```python
from build123d import *

# Parameters (mm, degrees)
BOX174_W                    = 2
BOX174_H                    = 6
BOX174_DEPTH                = 6
BOX175_W                    = 2
BOX175_H                    = 6
BOX175_DEPTH                = 6
BOX176_W                    = 2
BOX176_H                    = 6
BOX176_DEPTH                = 6
BOX173_W                    = 2
BOX173_H                    = 6
BOX173_DEPTH                = 6
CYLINDER397_R               = 1.5
CYLINDER397_DEPTH           = 100
CYLINDER398_R               = 1.5
CYLINDER398_DEPTH           = 100
CYLINDER395_R               = 1.5
CYLINDER395_DEPTH           = 100
CYLINDER396_R               = 1.5
CYLINDER396_DEPTH           = 100
CYLINDER375_R               = 1.5
CYLINDER375_DEPTH           = 50
CYLINDER375_PLACEMENT_ANGLE = 45
CYLINDER376_R               = 1.5
CYLINDER376_DEPTH           = 50
CYLINDER377_R               = 1.5
CYLINDER377_DEPTH           = 50
CYLINDER377_PLACEMENT_ANGLE = 135
CYLINDER378_R               = 1.5
CYLINDER378_DEPTH           = 50
CYLINDER379_R               = 1.5
CYLINDER379_DEPTH           = 50
CYLINDER379_PLACEMENT_ANGLE = 225
CYLINDER380_R               = 1.5
CYLINDER380_DEPTH           = 50
CYLINDER381_R               = 1.5
CYLINDER381_DEPTH           = 50
CYLINDER381_PLACEMENT_ANGLE = 45
CYLINDER374_R               = 1.5
CYLINDER374_DEPTH           = 50
BOX158_W                    = 8
BOX158_H                    = 6
BOX158_DEPTH                = 2
BOX158_PLACEMENT_ANGLE      = 45
BOX159_W                    = 8
BOX159_H                    = 6
BOX159_DEPTH                = 2
BOX160_W                    = 8
BOX160_H                    = 6
BOX160_DEPTH                = 2
BOX160_PLACEMENT_ANGLE      = 135
BOX161_W                    = 8
BOX161_H                    = 6
BOX161_DEPTH                = 2
BOX162_W                    = 8
BOX162_H                    = 6
BOX162_DEPTH                = 2
BOX162_PLACEMENT_ANGLE      = 225
BOX163_W                    = 8
BOX163_H                    = 6
BOX163_DEPTH                = 2
BOX164_W                    = 8
BOX164_H                    = 6
BOX164_DEPTH                = 2
BOX164_PLACEMENT_ANGLE      = 45
BOX157_W                    = 8
BOX157_H                    = 6
BOX157_DEPTH                = 2
CYLINDER006_R               = 3.5
CYLINDER006_DEPTH           = 16
TORUS004_R                  = 3.1
TUBE002_R                   = 54
TUBE002_R_2                 = 47
TUBE002_DEPTH               = 25


with BuildPart() as krychle174:
    # Box174 → Box174 (new body)
    with BuildSketch(Plane(origin=(32, -54, 24), x_dir=(1, 0, 0), z_dir=(0, 0, 1))):
        with Locations((1, 3)):
            Rectangle(BOX174_W, BOX174_H)
    extrude(amount=BOX174_DEPTH)


with BuildPart() as krychle175:
    # Box175 → Box175 (new body)
    with BuildSketch(Plane(origin=(38, 33, 39), x_dir=(1, 0, 0), z_dir=(0, 0, 1))):
        with Locations((1, 3)):
            Rectangle(BOX175_W, BOX175_H)
    extrude(amount=BOX175_DEPTH)


with BuildPart() as krychle176:
    # Box176 → Box176 (new body)
    with BuildSketch(Plane(origin=(38, -39, 39), x_dir=(1, 0, 0), z_dir=(0, 0, 1))):
        with Locations((1, 3)):
            Rectangle(BOX176_W, BOX176_H)
    extrude(amount=BOX176_DEPTH)


with BuildPart() as compound302:
    # Box173 → Box173 (new body)
    with BuildSketch(Plane(origin=(32, 48, 24), x_dir=(1, 0, 0), z_dir=(0, 0, 1))):
        with Locations((1, 3)):
            Rectangle(BOX173_W, BOX173_H)
    extrude(amount=BOX173_DEPTH)

    # Compound302: union Krychle174, Krychle175, Krychle176
    add(krychle174.part)
    add(krychle175.part)
    add(krychle176.part)


with BuildPart() as obj1:
    # Cylinder397 → Cylinder397 (new body)
    with BuildSketch(Plane(origin=(24, -51, 27), x_dir=(0, 0, -1), z_dir=(1, 0, 0))):
        Circle(CYLINDER397_R)
    extrude(amount=CYLINDER397_DEPTH)


with BuildPart() as obj2:
    # Cylinder398 → Cylinder398 (new body)
    with BuildSketch(Plane(origin=(34, 36, 42), x_dir=(0, 0, -1), z_dir=(1, 0, 0))):
        Circle(CYLINDER398_R)
    extrude(amount=CYLINDER398_DEPTH)


with BuildPart() as obj3:
    # Cylinder395 → Cylinder395 (new body)
    with BuildSketch(Plane(origin=(34, -36, 42), x_dir=(0, 0, -1), z_dir=(1, 0, 0))):
        Circle(CYLINDER395_R)
    extrude(amount=CYLINDER395_DEPTH)


with BuildPart() as compound303:
    # Cylinder396 → Cylinder396 (new body)
    with BuildSketch(Plane(origin=(24, 51, 27), x_dir=(0, 0, -1), z_dir=(1, 0, 0))):
        Circle(CYLINDER396_R)
    extrude(amount=CYLINDER396_DEPTH)

    # Compound303: union obj1, obj2, obj3
    add(obj1.part)
    add(obj2.part)
    add(obj3.part)


with BuildPart() as obj4:
    # Cylinder375 → Cylinder375 (new body)
    with BuildSketch(Plane.XY):
        Circle(CYLINDER375_R)
    extrude(amount=CYLINDER375_DEPTH)


with BuildPart() as obj4_1:
    # Cylinder375 placement: moved
    add(obj4.part.moved(Location((35.355339, 35.355339, -15))).rotate(Axis((35.355339, 35.355339, -15), (0, 0, 1)), CYLINDER375_PLACEMENT_ANGLE))


with BuildPart() as obj5:
    # Cylinder376 → Cylinder376 (new body)
    with BuildSketch(Plane(origin=(0, 50, -15), x_dir=(0, 1, 0), z_dir=(0, 0, 1))):
        Circle(CYLINDER376_R)
    extrude(amount=CYLINDER376_DEPTH)


with BuildPart() as obj6:
    # Cylinder377 → Cylinder377 (new body)
    with BuildSketch(Plane.XY):
        Circle(CYLINDER377_R)
    extrude(amount=CYLINDER377_DEPTH)


with BuildPart() as obj6_1:
    # Cylinder377 placement: moved
    add(obj6.part.moved(Location((-35.355339, 35.355339, -15))).rotate(Axis((-35.355339, 35.355339, -15), (0, 0, 1)), CYLINDER377_PLACEMENT_ANGLE))


with BuildPart() as obj7:
    # Cylinder378 → Cylinder378 (new body)
    with BuildSketch(Plane(origin=(-50, 0, -15), x_dir=(-1, 0, 0), z_dir=(0, 0, 1))):
        Circle(CYLINDER378_R)
    extrude(amount=CYLINDER378_DEPTH)


with BuildPart() as obj8:
    # Cylinder379 → Cylinder379 (new body)
    with BuildSketch(Plane.XY):
        Circle(CYLINDER379_R)
    extrude(amount=CYLINDER379_DEPTH)


with BuildPart() as obj8_1:
    # Cylinder379 placement: moved
    add(obj8.part.moved(Location((-35.355339, -35.355339, -15))).rotate(Axis((-35.355339, -35.355339, -15), (0, 0, 1)), CYLINDER379_PLACEMENT_ANGLE))


with BuildPart() as obj9:
    # Cylinder380 → Cylinder380 (new body)
    with BuildSketch(Plane(origin=(0, -50, -15), x_dir=(0, -1, 0), z_dir=(0, 0, 1))):
        Circle(CYLINDER380_R)
    extrude(amount=CYLINDER380_DEPTH)


with BuildPart() as obj10:
    # Cylinder381 → Cylinder381 (new body)
    with BuildSketch(Plane.XY):
        Circle(CYLINDER381_R)
    extrude(amount=CYLINDER381_DEPTH)


with BuildPart() as obj10_1:
    # Cylinder381 placement: moved
    add(obj10.part.moved(Location((35.355339, -35.355339, -15))).rotate(Axis((35.355339, -35.355339, -15), (0, 0, -1)), CYLINDER381_PLACEMENT_ANGLE))


with BuildPart() as compound298:
    # Cylinder374 → Cylinder374 (new body)
    with BuildSketch(Plane(origin=(50, 0, -15), x_dir=(1, 0, 0), z_dir=(0, 0, 1))):
        Circle(CYLINDER374_R)
    extrude(amount=CYLINDER374_DEPTH)

    # Compound298: union obj4, obj5, obj6, obj7, obj8, obj9, obj10
    add(obj4_1.part)
    add(obj5.part)
    add(obj6_1.part)
    add(obj7.part)
    add(obj8_1.part)
    add(obj9.part)
    add(obj10_1.part)


with BuildPart() as compound298_1:
    # Compound298 placement: moved
    add(compound298.part.moved(Location((0, 0, -5))))


with BuildPart() as krychle158:
    # Box158 → Box158 (new body)
    with BuildSketch(Plane.XY):
        with Locations((4, 3)):
            Rectangle(BOX158_W, BOX158_H)
    extrude(amount=BOX158_DEPTH)


with BuildPart() as krychle158_1:
    # Box158 placement: moved
    add(krychle158.part.moved(Location((34.648232, 30.405592, 23))).rotate(Axis((34.648232, 30.405592, 23), (0, 0, 1)), BOX158_PLACEMENT_ANGLE))


with BuildPart() as krychle159:
    # Box159 → Box159 (new body)
    with BuildSketch(Plane(origin=(3, 46, 23), x_dir=(0, 1, 0), z_dir=(0, 0, 1))):
        with Locations((4, 3)):
            Rectangle(BOX159_W, BOX159_H)
    extrude(amount=BOX159_DEPTH)


with BuildPart() as krychle160:
    # Box160 → Box160 (new body)
    with BuildSketch(Plane.XY):
        with Locations((4, 3)):
            Rectangle(BOX160_W, BOX160_H)
    extrude(amount=BOX160_DEPTH)


with BuildPart() as krychle160_1:
    # Box160 placement: moved
    add(krychle160.part.moved(Location((-30.405592, 34.648232, 23))).rotate(Axis((-30.405592, 34.648232, 23), (0, 0, 1)), BOX160_PLACEMENT_ANGLE))


with BuildPart() as krychle161:
    # Box161 → Box161 (new body)
    with BuildSketch(Plane(origin=(-46, 3, 23), x_dir=(-1, 0, 0), z_dir=(0, 0, 1))):
        with Locations((4, 3)):
            Rectangle(BOX161_W, BOX161_H)
    extrude(amount=BOX161_DEPTH)


with BuildPart() as krychle162:
    # Box162 → Box162 (new body)
    with BuildSketch(Plane.XY):
        with Locations((4, 3)):
            Rectangle(BOX162_W, BOX162_H)
    extrude(amount=BOX162_DEPTH)


with BuildPart() as krychle162_1:
    # Box162 placement: moved
    add(krychle162.part.moved(Location((-34.648232, -30.405592, 23))).rotate(Axis((-34.648232, -30.405592, 23), (0, 0, 1)), BOX162_PLACEMENT_ANGLE))


with BuildPart() as krychle163:
    # Box163 → Box163 (new body)
    with BuildSketch(Plane(origin=(-3, -46, 23), x_dir=(0, -1, 0), z_dir=(0, 0, 1))):
        with Locations((4, 3)):
            Rectangle(BOX163_W, BOX163_H)
    extrude(amount=BOX163_DEPTH)


with BuildPart() as krychle164:
    # Box164 → Box164 (new body)
    with BuildSketch(Plane.XY):
        with Locations((4, 3)):
            Rectangle(BOX164_W, BOX164_H)
    extrude(amount=BOX164_DEPTH)


with BuildPart() as krychle164_1:
    # Box164 placement: moved
    add(krychle164.part.moved(Location((30.405592, -34.648232, 23))).rotate(Axis((30.405592, -34.648232, 23), (0, 0, -1)), BOX164_PLACEMENT_ANGLE))


with BuildPart() as compound297:
    # Box157 → Box157 (new body)
    with BuildSketch(Plane(origin=(46, -3, 23), x_dir=(1, 0, 0), z_dir=(0, 0, 1))):
        with Locations((4, 3)):
            Rectangle(BOX157_W, BOX157_H)
    extrude(amount=BOX157_DEPTH)

    # Compound297: union Krychle158, Krychle159, Krychle160, Krychle161, Krychle162, Krychle163, Krychle164
    add(krychle158_1.part)
    add(krychle159.part)
    add(krychle160_1.part)
    add(krychle161.part)
    add(krychle162_1.part)
    add(krychle163.part)
    add(krychle164_1.part)


with BuildPart() as compound297_1:
    # Compound297 placement: moved
    add(compound297.part.moved(Location((0, 0, 1))))


with BuildPart() as obj11:
    # Cylinder006 → Cylinder006 (new body)
    with BuildSketch(Plane(origin=(-45.6, 0, 34), x_dir=(1, 0, 0), z_dir=(0, 0, 1))):
        Circle(CYLINDER006_R)
    extrude(amount=CYLINDER006_DEPTH)


with BuildPart() as obj12:
    # Torus004 → Torus004 (revolve)
    with BuildSketch(Plane(origin=(0, 0, 34), x_dir=(1, 0, 0), z_dir=(0, -1, 0))):
        with Locations((46.2, 0)):
            Circle(TORUS004_R)
    revolve(axis=Axis((0, 0, 34), (0, 0, 1)))


with BuildPart() as cut160:
    # Tube002 → Tube002 (new body)
    with BuildSketch(Plane.XY.offset(20)):
        Circle(TUBE002_R)
        Circle(TUBE002_R_2, mode=Mode.SUBTRACT)
    extrude(amount=TUBE002_DEPTH)

    # Cut009: cut obj12
    add(obj12.part, mode=Mode.SUBTRACT)

    # Cut010: cut obj11
    add(obj11.part, mode=Mode.SUBTRACT)

    # Cut151: cut Compound297
    add(compound297_1.part, mode=Mode.SUBTRACT)

    # Cut152: cut Compound298
    add(compound298_1.part, mode=Mode.SUBTRACT)

    # Cut159: cut Compound303
    add(compound303.part, mode=Mode.SUBTRACT)

    # Cut160: cut Compound302
    add(compound302.part, mode=Mode.SUBTRACT)


solid = cut160.part
```
Geometry: final body of the model. Coordinates: model frame, mm. A direction names the side the tool comes from. Coordinates: 2 decimals unless noted, no trailing zeros. Order: outer loops, then holes, each group sorted by start corner. A loop starts at its lowest first (then second) coordinate and runs counter-clockwise, first axis right, second up. Notation, with made-up numbers: (45, 86) -> (101, 86) arc R18 cw to (101, 105) -> close; hole circle Ø8 at (67.25, -18). An arc over 180 degrees is marked (long way). Write each question's results on one line, items separated by ' | '. Start each with the question number.
1) Cut plane B-B, the plane x = 0. State how many separate pieces and enclosed holes the cut face has, and give its area (3 significant figures).
2) Material intervals for line 1 along X through (y, z) = (0, 28.55); line 2 along X through (y, z) = (35.5, 28); line 3 along Z through (x, y) = (37, 36), sorted ascending.
3) First-contact query: pin 1 (4 mm diameter, centred on y = -36, z = 42, fed in from -X); pin 2 (1.6 mm diameter, centred on y = -35, z = 43.5, fed in from -X); pin 3 (4 mm diameter, centred on x = -6, z = 33.5, fed in from +Y); pin 4 (3 mm diameter, centred on x = -0.5, y = -49.5, fed in from -Z). Flat tips, straight axial feed; report the tip coordinate or a pass-through.
4) Mould query, pull axis Y, two halves, no side actions, for faces 1 (the flat face through (40, -34, 42)), 2 (the flat face through (-37, -37, 24)). Classes: released by +Y, released by -Y, zero draft, split by the parting line, or undercut.
5) Set-up query: faces 3 (the flat face through (50, 0, 30)), 4 (the flat face through (37, 37, 24)), 5 (the flat face through (52, 0, 24)), 6 (the cylindrical face through (36, 35.1, 43.2)). Return all of +Z, -Z, +X, -X, +Y, -Y with unobstructed straight access to the full face (end or side cutting, diameter ignored); none if empty.
6) Cut plane A-A, the plane z = 42. Output: boundary loops of the cut face in (x, y), and give its area (3 significant figures).
Checks:
1) separate pieces: 6 | enclosed holes: 0 | area: 254 mm^2
2) line 1: -54 to -51.5, -48.5 to -47, 47 to 48.5, 51.5 to 54 | line 2: -40.69 to -36.85, -33.86 to -30.8, 30.8 to 33.86, 36.85 to 40.69 | line 3: 20 to 24, 26 to 40.5, 43.5 to 45
3) pin 1: x = -41.95 | pin 2: x = -41.79 | pin 3: y = 53.85 | pin 4: z = 20
4) face 1: zero draft | face 2: undercut
5) face 3: -Z | face 4: none | face 5: +X, -X | face 6: +X
6) outline: (34, -37.5) -> (34, -34.5) -> (38, -34.5) -> (38, -33) -> (40, -33) -> (40, -34.5) -> (41.54, -34.5) arc R54 ccw to (41.54, 34.5) -> (40, 34.5) -> (40, 33) -> (38, 33) -> (38, 34.5) -> (34, 34.5) -> (34, 37.5) -> (38, 37.5) -> (38, 38.37) arc R54 ccw (long way) to (38, -38.37) -> (38, -37.5) -> close; hole (-46.89, -3.25) arc R47 ccw (long way) to (-46.89, 3.25) arc R3.5 ccw to start | area: 2,170 mm^2
